For this review, take the finished solid that the model builds, in its own axes (mm). A direction names the side the tool comes from. Give positions to 0.01 mm unless a question says otherwise; leave off trailing zeros. Write each loop counter-clockwise with the first axis right and the second up, starting at its lowest first coordinate (ties: lowest second). Pieces come first, ordered by that corner, then holes. Notation, with made-up numbers: M -30.75,66.25 L 14.25,66.25 A13 cw 14.25,82.25 Z; hole C -7.75,30 d10. An arc over 180 degrees is marked long. Write item = value, one per line.
```python
from build123d import *

# Parameters (mm, degrees)
EXTRUDE_THIN1_DEPTH     = 6.35
CUT_EXTRUDE1_DEPTH      = 23.3774
CUT_EXTRUDE1_DEPTH_BACK = 4.0226
SKETCH7_R               = 2.4
CUT_EXTRUDE3_DEPTH      = 4.0226
CUT_EXTRUDE2_DEPTH      = 15.9352
CUT_EXTRUDE2_DEPTH_BACK = 4.0226
SKETCH8_R               = 2.4
CUT_EXTRUDE4_DEPTH      = 4.0226


with BuildPart() as part:
    # Sketch4 → Extrude-Thin1 (new body, symmetric)
    with BuildSketch(Plane(origin=(0, 0, 0), x_dir=(1, 0, 0), z_dir=(0, 1, 0))):
        with BuildLine():
            Line((25.4, 0), (3.0226, 0))
            ThreePointArc((3.0226, 0), (0.885299043, -0.885299043), (0, -3.0226))
            Line((0, -3.0226), (0, -17.9578))
            Line((0, -17.9578), (3.0226, -17.9578))
            Line((3.0226, -17.9578), (3.0226, -3.0226))
            Line((3.0226, -3.0226), (25.4, -3.0226))
            Line((25.4, -3.0226), (25.4, 0))
        make_face()
    extrude(amount=EXTRUDE_THIN1_DEPTH, both=True)

    # Sketch5 → Cut-Extrude1 (cut, two sides)
    with BuildSketch(Plane(origin=(3.0226, 0, 0), x_dir=(0, 0, -1), z_dir=(1, 0, 0))) as cut_extrude1_sk:
        with BuildLine():
            Line((19.030404457, 42.52061468), (-15.4178, 6.35))
            ThreePointArc((-15.4178, 6.35), (-17.9578, 0), (-15.4178, -6.35))
            Line((-15.4178, -6.35), (19.030404457, -42.52061468))
            Line((19.030404457, -42.52061468), (-80.869388468, -42.52061468))
            Line((-80.869388468, -42.52061468), (-80.869388468, 42.52061468))
            Line((-80.869388468, 42.52061468), (19.030404457, 42.52061468))
        make_face()
    extrude(amount=CUT_EXTRUDE1_DEPTH, mode=Mode.SUBTRACT)
    extrude(cut_extrude1_sk.sketch, amount=-CUT_EXTRUDE1_DEPTH_BACK, mode=Mode.SUBTRACT)

    # Sketch7 → Cut-Extrude3 (cut, through all)
    with BuildSketch(Plane(origin=(3.0226, 0, 0), x_dir=(0, 0, -1), z_dir=(1, 0, 0))):
        with Locations((-10.0838, 0)):
            Circle(SKETCH7_R)
    extrude(amount=-CUT_EXTRUDE3_DEPTH, mode=Mode.SUBTRACT)

    # Sketch6 → Cut-Extrude2 (cut, two sides)
    with BuildSketch(Plane.XY.offset(3.0226)) as cut_extrude2_sk:
        with BuildLine():
            Line((-20.10675939, -51.46509736), (22.86, -6.35))
            ThreePointArc((22.86, -6.35), (25.4, 0), (22.86, 6.35))
            Line((22.86, 6.35), (-20.10675939, 51.46509736))
            Line((-20.10675939, 51.46509736), (104.496842842, 51.46509736))
            Line((104.496842842, 51.46509736), (104.496842842, -51.46509736))
            Line((104.496842842, -51.46509736), (-20.10675939, -51.46509736))
        make_face()
    extrude(amount=CUT_EXTRUDE2_DEPTH, mode=Mode.SUBTRACT)
    extrude(cut_extrude2_sk.sketch, amount=-CUT_EXTRUDE2_DEPTH_BACK, mode=Mode.SUBTRACT)

    # Sketch8 → Cut-Extrude4 (cut, through all)
    with BuildSketch(Plane.XY.offset(3.0226)):
        with Locations((16.5354, 0)):
            Circle(SKETCH8_R)
    extrude(amount=-CUT_EXTRUDE4_DEPTH, mode=Mode.SUBTRACT)


solid = part.part
```
1. For line 1 along Z through (x, y) = (22.5, -5.25); line 2 along Z through (x, y) = (1.5, 2), list the stretches that pass through material, from the lowest coordinate up. Write a range as from..to.
Responses:
line_1 = 0..3.02
line_2 = 0.41..8.76, 11.41..17.74
2. Machinability: for faces 4 (the face through (8, -6.35, 2.5)), 5 (the face through (14, -1, 3.023)), which of the approach directions +Z, -Z, +X, -X, +Y, -Y give a long, thin tool a straight path to every point of the face, cutting with its end or side? Answer none if there is none.
Responses:
face_4 = +Z, -Z, +X, -X, -Y
face_5 = +Z, +X, +Y, -Y
3. The part is to be moulded in two halves that separate along Z. For faces 1 (the face through (1.53, 0.11, 12.48)), 2 (the face through (8, 6.35, 2.5)), 3 (the face through (1.532, 0.098, 17.957)), say which applies: +Z half, -Z half, draft (parallel to the pull), parting line (faces both ways), or undercut.
Responses:
face_1 = undercut
face_2 = draft
face_3 = +Z half
4. We need section D-D, the plane y = 1.5. Write out the cut boundary in (x, z).
Responses:
outline = M 0,3.02 A3.02 ccw 3.02,0 L 14.66,0 L 14.66,3.02 L 3.02,3.02 L 3.02,8.21 L 0,8.21 Z; M 0,11.96 L 3.02,11.96 L 3.02,17.83 L 0,17.83 Z; M 18.41,0 L 25.28,0 L 25.28,3.02 L 18.41,3.02 Z
5. Insertion check: P1, Ø3, axis at x = 6.5, z = 8, coming from the +Y side; P2, Ø3, axis at y = -2, z = 3.5, coming from the +X side; P3, Ø1.5, axis at x = 18, y = -2, coming from the +Z side; P4, Ø6.5, axis at y = -1.5, z = 11.5, coming from the +X side. Each pin has a flat end and moves straight along its axis. Give the tip position at first contact, or say it passes through.
Responses:
P1 = through
P2 = 25.38
P3 = 3.02
P4 = 3.02
6. We need section A-A, the plane y = 0. Write out the cut boundary in (x, z), then the cut area to 3 significant figures.
Responses:
outline = M 0,3.02 A3.02 ccw 3.02,0 L 14.14,0 L 14.14,3.02 L 3.02,3.02 L 3.02,7.68 L 0,7.68 Z; M 0,12.48 L 3.02,12.48 L 3.02,17.96 L 0,17.96 Z; M 18.94,0 L 25.4,0 L 25.4,3.02 L 18.94,3.02 Z
area = 90.9 mm2
7. We need section B-B, the plane z = 11. Write out the cut boundary in (x, y), then the cut area to 3 significant figures.
Responses:
outline = M 0,-6.35 L 3.02,-6.35 L 3.02,-2.22 L 0,-2.22 Z; M 0,2.22 L 3.02,2.22 L 3.02,6.35 L 0,6.35 Z
area = 25.0 mm2
